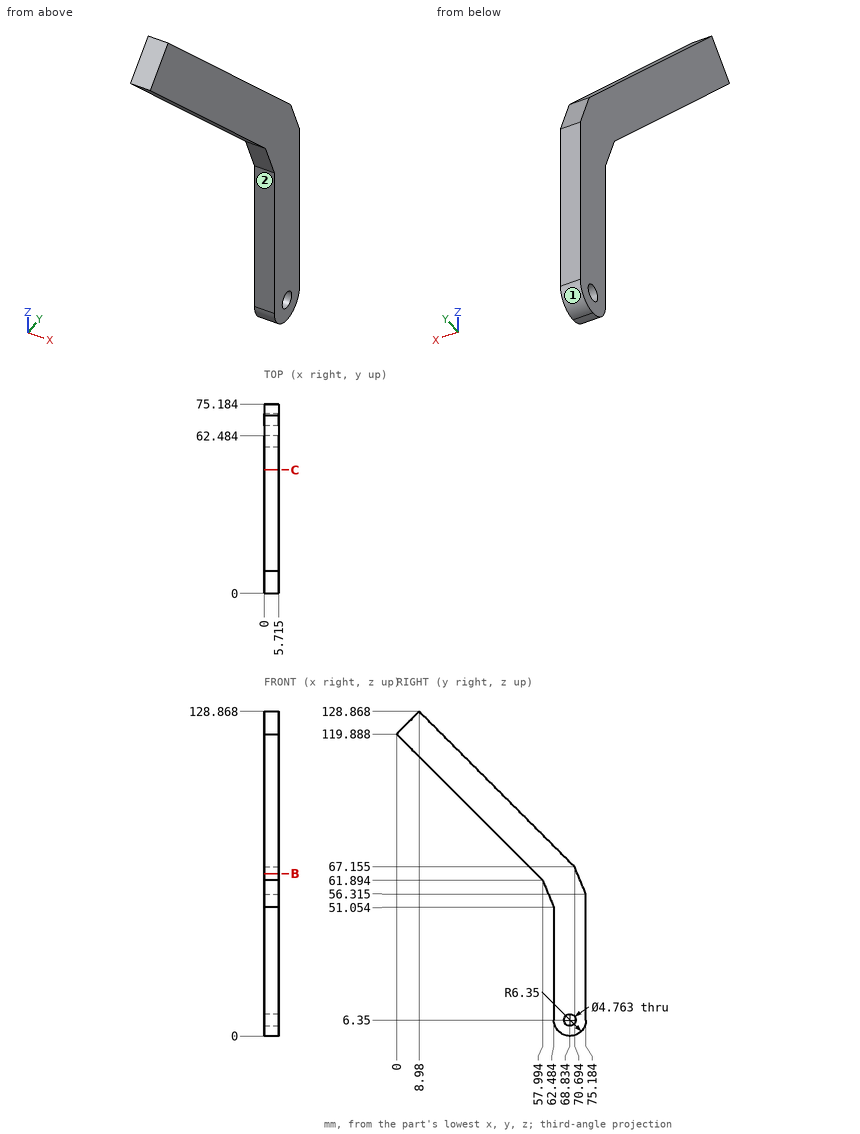
Design review of the part shown in the three views and the two pictorial views. Dimensions are in mm from the part's minimum x, y and z. A direction names the side the tool comes from. Round coordinates to 2 decimals unless told otherwise and drop trailing zeros. Write each loop counter-clockwise with the first axis right and the second up, starting at its lowest first coordinate (ties: lowest second). Pieces come first, ordered by that corner, then holes.
Item 1: Consider section C-C on y = 49. Give the boundary of the cut face in (x, z) (1 decimal).
Item 2: For the marked faces 1 and 2, list the 3-axis set-ups (+Z, -Z, +X, -X, +Y, -Y) from which the entire face can be reached by the end or side of a thin tool; tool diameter is ignored.
Item 3: Wall thickness on L1, parallel to Y at x = 5.4, z = 22.5 (1 decimal); L2, parallel to Z at x = 0.95, y = 6 (1 decimal): over which ranges is each line inside the solid? List them lowest first.
Item 4: For pin 1 Ø3 at (x, z) = (3.5, 39) entering from -Y; pin 2 Ø2 at (x, y) = (0.5, 66) entering from -Z; pin 3 Ø3 at (x, y) = (4.5, 42) entering from -Z, all flat-tipped, find the tip position at first contact; note any pin that passes through.
Item 5: Consider section B-B on z = 64.5. Give the boundary of the cut face in (x, y) (1 decimal).
Check values:
1. outline: (0, 70.9) - (5.7, 70.9) - (5.7, 88.8) - (0, 88.8) - close
2. face 1: -Z, +X, -X, +Y
2. face 2: -Z, +X, -X, -Y
3. L1: y = 62.5 to 75.2
3. L2: z = 113.9 to 125.9
4. pin 1: stops at y = 62.48
4. pin 2: stops at z = 0.27
4. pin 3: stops at z = 76.39
5. outline: (0, 55.4) - (5.7, 55.4) - (5.7, 71.8) - (0, 71.8) - close
